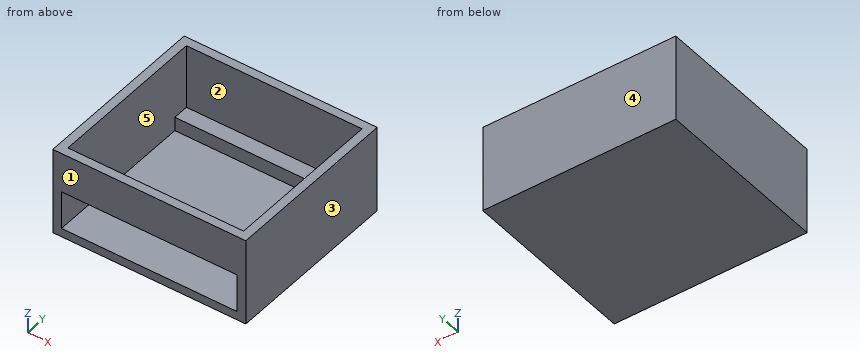
from build123d import *

# Parameters (mm, degrees)
SKETCH_1_W          = 111
SKETCH_1_H          = 102
SKETCH_1_W_2        = 101
SKETCH_1_H_2        = 92
EXTRUDE_1_DEPTH     = 45
SKETCH_2_W          = 111
SKETCH_2_H          = 102
EXTRUDE_2_DEPTH     = 5
SKETCH_3_W          = 101
SKETCH_3_H          = 22
CUT_EXTRUDE_4_DEPTH = 5
SKETCH_4_W          = 101
SKETCH_4_H          = 9
EXTRUDE_3_DEPTH     = 8


with BuildPart() as part:
    # 草圖1 → 填料-伸長1 (new body)
    with BuildSketch(Plane.XY):
        with Locations((-27.081120075, 1.427877732)):
            Rectangle(SKETCH_1_W, SKETCH_1_H)
        with Locations((-27.081120075, 1.427877732)):
            Rectangle(SKETCH_1_W_2, SKETCH_1_H_2, mode=Mode.SUBTRACT)
    extrude(amount=EXTRUDE_1_DEPTH)

    # 草圖2 → 填料-伸長2 (add)
    with BuildSketch(Plane(origin=(0, 0, 0), x_dir=(-1, 0, 0), z_dir=(0, 0, -1))):
        with Locations((27.081120075, 1.427877732)):
            Rectangle(SKETCH_2_W, SKETCH_2_H)
    extrude(amount=EXTRUDE_2_DEPTH)

    # 草圖3 → 除料-伸長4 (cut)
    with BuildSketch(Plane.XZ.offset(49.572122268)):
        with Locations((-27.081120075, 11)):
            Rectangle(SKETCH_3_W, SKETCH_3_H)
    extrude(amount=-CUT_EXTRUDE_4_DEPTH, mode=Mode.SUBTRACT)

    # 草圖4 → 填料-伸長3 (add)
    with BuildSketch(Plane.XY):
        with Locations((-27.081120075, 42.927877732)):
            Rectangle(SKETCH_4_W, SKETCH_4_H)
    extrude(amount=EXTRUDE_3_DEPTH)


solid = part.part
The model under review builds one solid part; all positions refer to its coordinate system, in mm. Face numbers are marked on the shaded views. A direction names the side the tool comes from. Coordinates: 2 decimals unless noted, no trailing zeros. Order: outer loops, then holes, each group sorted by start corner. A loop starts at its lowest first (then second) coordinate and runs counter-clockwise, first axis right, second up. Notation, with made-up numbers: (47, 8) -> (54, 8) arc R11 ccw to (54, 12) -> close; hole circle Ø6 at (26.5, 64). An arc over 180 degrees is marked (long way). Answer in a Markdown table with one row per item.
(1) Consider section D-D (z = 17). Write out the cut boundary in (x, y).
Answers:
| item | result |
|---|---|
| outline | (-82.58, -49.57) -> (-77.58, -49.57) -> (-77.58, 47.43) -> (23.42, 47.43) -> (23.42, -49.57) -> (28.42, -49.57) -> (28.42, 52.43) -> (-82.58, 52.43) -> close |
(2) Consider section B-B (z = 38). Write out the cut boundary in (x, y).
Answers:
| item | result |
|---|---|
| outline | (-82.58, -49.57) -> (28.42, -49.57) -> (28.42, 52.43) -> (-82.58, 52.43) -> close; hole (-77.58, -44.57) -> (23.42, -44.57) -> (23.42, 47.43) -> (-77.58, 47.43) -> close |
(3) Insertion check: pin 1 (2.5 mm diameter, centred on x = -11, z = 4, fed in from -Y); pin 2 (5 mm diameter, centred on x = -29, y = 0.5, fed in from +Z); pin 3 (4.5 mm diameter, centred on x = -23.5, y = 42, fed in from +Z). Each pin has a flat end and moves straight along its axis. Give the tip position at first contact, or say it passes through.
Answers:
| item | result |
|---|---|
| pin 1 | y = 38.43 |
| pin 2 | z = 0 |
| pin 3 | z = 8 |
(4) Machinability: for the marked faces 1 and 2, which of the approach directions +Z, -Z, +X, -X, +Y, -Y give a long, thin tool a straight path to every point of the face, cutting with its end or side? Answer none if there is none.
Answers:
| item | result |
|---|---|
| face 1 | +Z, -Z, +X, -X, -Y |
| face 2 | +Z |
(5) Consider section C-C (y = -30). Write out the cut boundary in (x, z).
Answers:
| item | result |
|---|---|
| outline | (-82.58, -5) -> (28.42, -5) -> (28.42, 45) -> (23.42, 45) -> (23.42, 0) -> (-77.58, 0) -> (-77.58, 45) -> (-82.58, 45) -> close |
(6) Wall thickness on line 1 along Y through (x, z) = (-49, 29); line 2 along X through (y, z) = (15.5, 7.5); line 3 along Y through (x, z) = (-63.5, 0.5): over which ranges is each line inside the solid? List them lowest first.
Answers:
| item | result |
|---|---|
| line 1 | -49.57 to -44.57, 47.43 to 52.43 |
| line 2 | -82.58 to -77.58, 23.42 to 28.42 |
| line 3 | 38.43 to 52.43 |
(7) Consider section A-A (x = -6.5). Write out the cut boundary in (y, z).
Answers:
| item | result |
|---|---|
| outline | (-49.57, -5) -> (52.43, -5) -> (52.43, 45) -> (47.43, 45) -> (47.43, 8) -> (38.43, 8) -> (38.43, 0) -> (-49.57, 0) -> close; (-49.57, 22) -> (-44.57, 22) -> (-44.57, 45) -> (-49.57, 45) -> close |
(8) The part is to be moulded in two halves that separate along X. For the marked faces 3, 4 and 5, say which applies: +X half, -X half, draft (parallel to the pull), parting line (faces both ways), or undercut.
Answers:
| item | result |
|---|---|
| face 3 | +X half |
| face 4 | draft |
| face 5 | undercut |
